Work out the finished part from the listing and answer in its coordinate system (mm). A direction names the side the tool comes from. Coordinates: 2 decimals unless noted, no trailing zeros. Loops run counter-clockwise (first coordinate to the right, second up) from the corner with the lowest first, then second, coordinate; pieces in that order, holes last. Notation, with made-up numbers: M 13.5,-5 L 44.5,-5 A19 ccw 44.5,12 Z; hole C -15.5,23.5 d9. An arc over 180 degrees is marked long. Write each question's results on one line, items separated by ' | '.
```python
from build123d import *
from OCP.BRepFilletAPI import BRepFilletAPI_MakeChamfer, BRepFilletAPI_MakeFillet

# Parameters (mm, degrees)
BOSS_EXTRU_1_DEPTH      = 15.5
BOSS_EXTRU_2_DEPTH      = 30
ESQUISSE2_R             = 1.6
ENL_V_MAT_EXTRU_1_DEPTH = 63.869786066
ESQUISSE3_R             = 2
ENL_V_MAT_EXTRU_2_DEPTH = 13
ESQUISSE9_R             = 2.5
ENL_V_MAT_EXTRU_7_DEPTH = 7
ENL_V_MAT_EXTRU_3_REACH = 64.87
ESQUISSE5_R             = 1.6
ESQUISSE6_R             = 2.1
ENL_V_MAT_EXTRU_4_DEPTH = 13
ESQUISSE10_R            = 2.5
ENL_V_MAT_EXTRU_8_DEPTH = 7
ENL_V_MAT_EXTRU_5_REACH = 65.759
ESQUISSE7_R             = 1.6
ESQUISSE8_R             = 2
ENL_V_MAT_EXTRU_6_DEPTH = 12.5
ESQUISSE11_R            = 2.5
ENL_V_MAT_EXTRU_9_DEPTH = 6.5
CONG_1_R1               = 2.5
CONG_1_R2               = 4
CONG_1_R3               = 9
CHANFREIN1_SIZE         = 3.2
CHANFREIN2_SIZE         = 1.2
CHANFREIN2_SIZE2        = 1.697056275


with BuildPart() as part:
    # Esquisse1 → Boss.-Extru.1 (new body)
    with BuildSketch(Plane(origin=(0, 0, 0), x_dir=(1, 0, 0), z_dir=(0, 1, 0))):
        with BuildLine():
            Line((-27.386127875, 7.5), (-60, 7.5))
            Line((-60, 7.5), (-60, -7.5))
            Line((-60, -7.5), (60, -7.5))
            Line((60, -7.5), (60, 7.5))
            Line((60, 7.5), (27.386127875, 7.5))
            ThreePointArc((27.386127875, 7.5), (0, -2.5), (-27.386127875, 7.5))
        make_face()
    extrude(amount=BOSS_EXTRU_1_DEPTH)

    # Esquisse12 → Boss.-Extru.2 (add, symmetric)
    with BuildSketch(Plane(origin=(0, 0, 0), x_dir=(0, 0, -1), z_dir=(1, 0, 0))):
        Polygon((-7.5, 0), (-10.6, 0), (-10.6, 6), (-9, 6), (-9, 2), (-7.5, 2), align=None)
    extrude(amount=BOSS_EXTRU_2_DEPTH, both=True)

    # Esquisse2 → Enlèv. mat.-Extru.1 (cut, through all)
    with BuildSketch(Plane(origin=(0, 15.5, 0), x_dir=(1, 0, 0), z_dir=(0, 1, 0))):
        with Locations(Location((45, 2.5, 0), (0, 0, 270))):
            Circle(ESQUISSE2_R)
    enl_v_mat_extru_1 = extrude(amount=-ENL_V_MAT_EXTRU_1_DEPTH, mode=Mode.SUBTRACT)

    # Esquisse3 → Enlèv. mat.-Extru.2 (cut)
    with BuildSketch(Plane.XZ):
        with Locations(Location((45, -2.5, 0), (0, 0, 270))):
            Circle(ESQUISSE3_R)
    enl_v_mat_extru_2 = extrude(amount=-ENL_V_MAT_EXTRU_2_DEPTH, mode=Mode.SUBTRACT)

    # Esquisse9 → Enlèv. mat.-Extru.7 (cut)
    with BuildSketch(Plane.XZ):
        with Locations(Location((45, -2.5, 0), (0, 0, 270))):
            Circle(ESQUISSE9_R)
    enl_v_mat_extru_7 = extrude(amount=-ENL_V_MAT_EXTRU_7_DEPTH, mode=Mode.SUBTRACT)

    # Esquisse5 → Enlèv. mat.-Extru.3 (cut, up to next)
    with BuildSketch(Plane.XZ, mode=Mode.PRIVATE) as enl_v_mat_extru_3_sk1:
        with Locations(Location((40, 2.5, 0), (0, 0, 270))):
            Circle(ESQUISSE5_R)
    enl_v_mat_extru_3_tool1 = extrude(enl_v_mat_extru_3_sk1.sketch, amount=-ENL_V_MAT_EXTRU_3_REACH, mode=Mode.PRIVATE) & part.part
    enl_v_mat_extru_3 = enl_v_mat_extru_3_tool1.solids().sort_by_distance((40, 0, 2.5))[0]
    add(enl_v_mat_extru_3, mode=Mode.SUBTRACT)

    # Esquisse6 → Enlèv. mat.-Extru.4 (cut)
    with BuildSketch(Plane(origin=(0, 15.5, 0), x_dir=(1, 0, 0), z_dir=(0, 1, 0))):
        with Locations(Location((40, -2.5, 0), (0, 0, 270))):
            Circle(ESQUISSE6_R)
    enl_v_mat_extru_4 = extrude(amount=-ENL_V_MAT_EXTRU_4_DEPTH, mode=Mode.SUBTRACT)

    # Esquisse10 → Enlèv. mat.-Extru.8 (cut)
    with BuildSketch(Plane(origin=(0, 15.5, 0), x_dir=(1, 0, 0), z_dir=(0, 1, 0))):
        with Locations(Location((40, -2.5, 0), (0, 0, 270))):
            Circle(ESQUISSE10_R)
    enl_v_mat_extru_8 = extrude(amount=-ENL_V_MAT_EXTRU_8_DEPTH, mode=Mode.SUBTRACT)

    # Esquisse7 → Enlèv. mat.-Extru.5 (cut, up to next)
    with BuildSketch(Plane.XY.offset(7.5), mode=Mode.PRIVATE) as enl_v_mat_extru_5_sk1:
        with Locations((35, 7)):
            Circle(ESQUISSE7_R)
    enl_v_mat_extru_5_tool1 = extrude(enl_v_mat_extru_5_sk1.sketch, amount=-ENL_V_MAT_EXTRU_5_REACH, mode=Mode.PRIVATE) & part.part
    enl_v_mat_extru_5 = enl_v_mat_extru_5_tool1.solids().sort_by_distance((35, 7, 7.5))[0]
    add(enl_v_mat_extru_5, mode=Mode.SUBTRACT)

    # Esquisse8 → Enlèv. mat.-Extru.6 (cut)
    with BuildSketch(Plane(origin=(0, 0, -7.5), x_dir=(-1, 0, 0), z_dir=(0, 0, -1))):
        with Locations((-35, 7)):
            Circle(ESQUISSE8_R)
    enl_v_mat_extru_6 = extrude(amount=-ENL_V_MAT_EXTRU_6_DEPTH, mode=Mode.SUBTRACT)

    # Esquisse11 → Enlèv. mat.-Extru.9 (cut)
    with BuildSketch(Plane(origin=(0, 0, -7.5), x_dir=(-1, 0, 0), z_dir=(0, 0, -1))):
        with Locations((-35, 7)):
            Circle(ESQUISSE11_R)
    enl_v_mat_extru_9 = extrude(amount=-ENL_V_MAT_EXTRU_9_DEPTH, mode=Mode.SUBTRACT)

    # Symétrie1: Enlèv. mat.-Extru.1, Enlèv. mat.-Extru.2, Enlèv. mat.-Extru.7, Enlèv. mat.-Extru.3, Enlèv. mat.-Extru.4, Enlèv. mat.-Extru.8, Enlèv. mat.-Extru.5, Enlèv. mat.-Extru.6, Enlèv. mat.-Extru.9 across plane
    add(enl_v_mat_extru_1.mirror(Plane(origin=(0, 0, 0), x_dir=(0, 0, 1), z_dir=(1, 0, 0))), mode=Mode.SUBTRACT)
    add(enl_v_mat_extru_2.mirror(Plane(origin=(0, 0, 0), x_dir=(0, 0, 1), z_dir=(1, 0, 0))), mode=Mode.SUBTRACT)
    add(enl_v_mat_extru_7.mirror(Plane(origin=(0, 0, 0), x_dir=(0, 0, 1), z_dir=(1, 0, 0))), mode=Mode.SUBTRACT)
    add(enl_v_mat_extru_3.mirror(Plane(origin=(0, 0, 0), x_dir=(0, 0, 1), z_dir=(1, 0, 0))), mode=Mode.SUBTRACT)
    add(enl_v_mat_extru_4.mirror(Plane(origin=(0, 0, 0), x_dir=(0, 0, 1), z_dir=(1, 0, 0))), mode=Mode.SUBTRACT)
    add(enl_v_mat_extru_8.mirror(Plane(origin=(0, 0, 0), x_dir=(0, 0, 1), z_dir=(1, 0, 0))), mode=Mode.SUBTRACT)
    add(enl_v_mat_extru_5.mirror(Plane(origin=(0, 0, 0), x_dir=(0, 0, 1), z_dir=(1, 0, 0))), mode=Mode.SUBTRACT)
    add(enl_v_mat_extru_6.mirror(Plane(origin=(0, 0, 0), x_dir=(0, 0, 1), z_dir=(1, 0, 0))), mode=Mode.SUBTRACT)
    add(enl_v_mat_extru_9.mirror(Plane(origin=(0, 0, 0), x_dir=(0, 0, 1), z_dir=(1, 0, 0))), mode=Mode.SUBTRACT)

    # Congé1: one fillet with a radius per group of edges: ONE call of the kernel's fillet builder (fillet() takes one radius for all edges)
    cong_1_edges_1 = [part.edges().sort_by_distance(p)[0] for p in [
        (27.386127875, 7.75, -7.5),
        (-27.386127875, 7.75, -7.5),
    ]]
    cong_1_edges_2 = [part.edges().sort_by_distance(p)[0] for p in [
        (60, 7.75, -7.5),
        (-60, 7.75, -7.5),
    ]]
    cong_1_edges_3 = [part.edges().sort_by_distance(p)[0] for p in [
        (60, 7.75, 7.5),
        (-60, 7.75, 7.5),
    ]]
    cong_1 = BRepFilletAPI_MakeFillet(part.part.solid().wrapped)
    for e in cong_1_edges_1:
        cong_1.Add(CONG_1_R1, e.wrapped)
    for e in cong_1_edges_2:
        cong_1.Add(CONG_1_R2, e.wrapped)
    for e in cong_1_edges_3:
        cong_1.Add(CONG_1_R3, e.wrapped)
    add(Compound.cast(cong_1.Shape()), mode=Mode.REPLACE)

    # Chanfrein1
    # the kernel refuses this chamfer: 3.2 mm, written as the material it adds along each edge
    with BuildSketch(Plane(origin=(30, 10.229385561, 7.5), x_dir=(0.9996219169112968, 0, -0.027495876610586226), z_dir=(0, -1, 0))) as chanfrein1_piece_1_section:
        Polygon((CHANFREIN1_SIZE * 0.999621916911, CHANFREIN1_SIZE * 0.0274958766106), (-CHANFREIN1_SIZE * 0.0274958766106, CHANFREIN1_SIZE * 0.999621916911), (0, 0), align=None)
    chanfrein1_piece_1 = extrude(amount=10.229385561, mode=Mode.PRIVATE)
    chanfrein1_piece_1 = split(chanfrein1_piece_1, bisect_by=Plane(origin=(30.510820254, 2, 9.595713626), z_dir=(0, 1, 0)), keep=Keep.TOP, mode=Mode.PRIVATE)
    chanfrein1_piece_1 = split(chanfrein1_piece_1, bisect_by=Plane(origin=(30.510820254, 4, 10.6), z_dir=(0, 0, -1)), keep=Keep.TOP, mode=Mode.PRIVATE)
    chanfrein1_piece_1 = split(chanfrein1_piece_1, bisect_by=Plane(origin=(30.510820254, 6, 9.595713626), z_dir=(0, -1, 0)), keep=Keep.TOP, mode=Mode.PRIVATE)
    chanfrein1_piece_1 = split(chanfrein1_piece_1, bisect_by=Plane(origin=(30.510820254, 4, 9), z_dir=(0, 0, 1)), keep=Keep.TOP, mode=Mode.PRIVATE)
    add(chanfrein1_piece_1)
    with BuildSketch(Plane(origin=(30, 2, 7.5), x_dir=(0.9996219169112966, 0, -0.02749587661058616), z_dir=(0, -1, 0))) as chanfrein1_piece_2_section:
        Polygon((CHANFREIN1_SIZE * 0.999621916911, CHANFREIN1_SIZE * 0.0274958766106), (-CHANFREIN1_SIZE * 0.0274958766106, CHANFREIN1_SIZE * 0.999621916911), (0, 0), align=None)
    chanfrein1_piece_2 = extrude(amount=2, mode=Mode.PRIVATE)
    chanfrein1_piece_2 = split(chanfrein1_piece_2, bisect_by=Plane(origin=(31.278670845, 1, 9), z_dir=(0, 0, -1)), keep=Keep.TOP, mode=Mode.PRIVATE)
    add(chanfrein1_piece_2)
    with BuildSketch(Plane(origin=(30, 2, 7.5), x_dir=(0.9996219169112966, 0, -0.02749587661058616), z_dir=(0, -1, 0))) as chanfrein1_piece_3_section:
        Polygon((CHANFREIN1_SIZE * 0.999621916911, CHANFREIN1_SIZE * 0.0274958766106), (-CHANFREIN1_SIZE * 0.0274958766106, CHANFREIN1_SIZE * 0.999621916911), (0, 0), align=None)
    chanfrein1_piece_3 = extrude(amount=2, mode=Mode.PRIVATE)
    chanfrein1_piece_3 = split(chanfrein1_piece_3, bisect_by=Plane(origin=(30.510820254, 1, 10.6), z_dir=(0, 0, -1)), keep=Keep.TOP, mode=Mode.PRIVATE)
    chanfrein1_piece_3 = split(chanfrein1_piece_3, bisect_by=Plane(origin=(30.510820254, 1, 9), z_dir=(0, 0, 1)), keep=Keep.TOP, mode=Mode.PRIVATE)
    add(chanfrein1_piece_3)
    with BuildSketch(Plane(origin=(-30, 10.229385561, 7.5), x_dir=(-0.9996219169112968, 0, -0.027495876610586226), z_dir=(0, -1, 0))) as chanfrein1_piece_4_section:
        Polygon((CHANFREIN1_SIZE * 0.999621916911, -CHANFREIN1_SIZE * 0.0274958766106), (-CHANFREIN1_SIZE * 0.0274958766106, -CHANFREIN1_SIZE * 0.999621916911), (0, 0), align=None)
    chanfrein1_piece_4 = extrude(amount=10.229385561, mode=Mode.PRIVATE)
    chanfrein1_piece_4 = split(chanfrein1_piece_4, bisect_by=Plane(origin=(-30.510820254, 2, 9.595713626), z_dir=(0, 1, 0)), keep=Keep.TOP, mode=Mode.PRIVATE)
    chanfrein1_piece_4 = split(chanfrein1_piece_4, bisect_by=Plane(origin=(-30.510820254, 4, 10.6), z_dir=(0, 0, -1)), keep=Keep.TOP, mode=Mode.PRIVATE)
    chanfrein1_piece_4 = split(chanfrein1_piece_4, bisect_by=Plane(origin=(-30.510820254, 6, 9.595713626), z_dir=(0, -1, 0)), keep=Keep.TOP, mode=Mode.PRIVATE)
    chanfrein1_piece_4 = split(chanfrein1_piece_4, bisect_by=Plane(origin=(-30.510820254, 4, 9), z_dir=(0, 0, 1)), keep=Keep.TOP, mode=Mode.PRIVATE)
    add(chanfrein1_piece_4)
    with BuildSketch(Plane(origin=(-30, 2, 7.5), x_dir=(-0.9996219169112968, 0, -0.027495876610586226), z_dir=(0, -1, 0))) as chanfrein1_piece_5_section:
        Polygon((CHANFREIN1_SIZE * 0.999621916911, -CHANFREIN1_SIZE * 0.0274958766106), (-CHANFREIN1_SIZE * 0.0274958766106, -CHANFREIN1_SIZE * 0.999621916911), (0, 0), align=None)
    chanfrein1_piece_5 = extrude(amount=2, mode=Mode.PRIVATE)
    chanfrein1_piece_5 = split(chanfrein1_piece_5, bisect_by=Plane(origin=(-31.278670845, 1, 9), z_dir=(0, 0, -1)), keep=Keep.TOP, mode=Mode.PRIVATE)
    add(chanfrein1_piece_5)
    with BuildSketch(Plane(origin=(-30, 2, 7.5), x_dir=(-0.9996219169112968, 0, -0.027495876610586226), z_dir=(0, -1, 0))) as chanfrein1_piece_6_section:
        Polygon((CHANFREIN1_SIZE * 0.999621916911, -CHANFREIN1_SIZE * 0.0274958766106), (-CHANFREIN1_SIZE * 0.0274958766106, -CHANFREIN1_SIZE * 0.999621916911), (0, 0), align=None)
    chanfrein1_piece_6 = extrude(amount=2, mode=Mode.PRIVATE)
    chanfrein1_piece_6 = split(chanfrein1_piece_6, bisect_by=Plane(origin=(-30.510820254, 1, 10.6), z_dir=(0, 0, -1)), keep=Keep.TOP, mode=Mode.PRIVATE)
    chanfrein1_piece_6 = split(chanfrein1_piece_6, bisect_by=Plane(origin=(-30.510820254, 1, 9), z_dir=(0, 0, 1)), keep=Keep.TOP, mode=Mode.PRIVATE)
    add(chanfrein1_piece_6)

    # Chanfrein2: one chamfer whose edges measure the first distance from different faces: ONE call of the kernel's chamfer builder (chamfer() names one face for all edges)
    chanfrein2_edges_1 = [part.edges().sort_by_distance(p)[0] for p in [
        (31.7, 4, 9),
    ]]
    chanfrein2_side_1 = [part.faces().sort_by_distance(p)[0] for p in [
        (31.269047619, 2.523809524, 9.430952381),
    ]]
    chanfrein2_edges_2 = [part.edges().sort_by_distance(p)[0] for p in [
        (-31.7, 4, 9),
    ]]
    chanfrein2_side_2 = [part.faces().sort_by_distance(p)[0] for p in [
        (-31.269047619, 2.523809524, 9.430952381),
    ]]
    chanfrein2 = BRepFilletAPI_MakeChamfer(part.part.solid().wrapped)
    for e in chanfrein2_edges_1:
        chanfrein2.Add(CHANFREIN2_SIZE, CHANFREIN2_SIZE2, e.wrapped, chanfrein2_side_1[0].wrapped)  # the first distance lies on this face
    for e in chanfrein2_edges_2:
        chanfrein2.Add(CHANFREIN2_SIZE, CHANFREIN2_SIZE2, e.wrapped, chanfrein2_side_2[0].wrapped)  # the first distance lies on this face
    add(Compound.cast(chanfrein2.Shape()), mode=Mode.REPLACE)


solid = part.part
```
1) Straight lines are drawn through the part: probe 1 along Y at (x, z) = (-35, -6); probe 2 along X at (y, z) = (11.25, -2); probe 3 along X at (y, z) = (3.75, -2.5). For each, find the intervals that lie inside material, in ascending order. Write a range as [from, to].
Check result:
probe 1: [0, 4.5], [9.5, 15.5] | probe 2: [-60, -46.94], [-43.06, -19.03], [19.03, 43.06], [46.94, 60] | probe 3: [-60, -47.5], [-42.5, -20], [20, 42.5], [47.5, 60]
2) Which of the six approach directions +Z, -Z, +X, -X, +Y, -Y give full straight-line access (tool end or side, diameter ignored) to faces 1 (the face through (44, 13, -1)), 2 (the face through (-33.092, 7.601, 1.958)), 3 (the face through (37.56, 12.05, 1.96))?
Check result:
face 1: -Y | face 2: -Z | face 3: +Y
3) Find section B-B, the plane y = 3.5. Give the vertices of the cut face in (x, z).
Check result:
outline: M -60,-3.5 A4 ccw -56,-7.5 L -28.28,-7.5 A2.5 ccw -26.71,-6.94 A42.5 cw 26.71,-6.94 A2.5 ccw 28.28,-7.5 L 56,-7.5 A4 ccw 60,-3.5 L 60,-1.5 A9 ccw 51,7.5 L -51,7.5 A9 ccw -60,-1.5 Z; M -30.85,9.85 L -30,9 L 30,9 L 30.85,9.85 L 30.1,10.6 L -30.1,10.6 Z; hole C -45,-2.5 d5; hole C -40,2.5 d4.2; hole C 40,2.5 d4.2; hole C 45,-2.5 d5
4) Find section D-D, the plane x = -45. Give the vertices of the cut face in (y, z).
Check result:
outline: M 0,-7.5 L 15.5,-7.5 L 15.5,-4.1 L 13,-4.1 L 13,-4.5 L 7,-4.5 L 7,-5 L 0,-5 Z; M 0,0 L 7,0 L 7,-0.5 L 13,-0.5 L 13,-0.9 L 15.5,-0.9 L 15.5,7.5 L 0,7.5 Z
5) For a pull along Z with two mould halves and no side action, classify faces 4 (the face through (0, 2, 8)), 5 (the face through (-32.69, 6.04, -4.3)), 6 (the face through (58.797, 7.858, -6.359)) as released by +Z, released by -Z, zero draft, split by the parting line, or undercut.
Check result:
face 4: undercut | face 5: zero draft | face 6: released by -Z
6) Given pin 1 Ø6 at (x, y) = (19.5, 2.5) entering from -Z; pin 2 Ø2.5 at (x, y) = (35, 6.5) entering from -Z; pin 3 Ø2.5 at (x, z) = (-44, -3) entering from -Y, each flat-ended and moving along its own axis, determine where each tip first touches the part or whether it passes through.
Check result:
pin 1: z = -3.94 | pin 2: z = 5 | pin 3: y = 7
7) Find section A-A, the plane z = -2.5. Give the number of separate pieces and of enclosed holes in the cut face, and give its area (3 significant figures).
Check result:
separate pieces: 4 | enclosed holes: 2 | area: 1,070 mm^2
8) Find section C-C, the plane x = 35. Give the vertices of the cut face in (y, z), and give its area (3 significant figures).
Check result:
outline: M 0,-7.5 L 4.5,-7.5 L 4.5,-1 L 5,-1 L 5,5 L 5.4,5 L 5.4,7.5 L 0,7.5 Z; M 8.6,5 L 9,5 L 9,-1 L 9.5,-1 L 9.5,-7.5 L 15.5,-7.5 L 15.5,7.5 L 8.6,7.5 Z | area: 168 mm^2
